from build123d import *

# Parameters (mm, degrees)
SKETCH2_R                = 3
BOSS_EXTRUDE1_DEPTH      = 20.5
BOSS_EXTRUDE1_DEPTH_BACK = 20.5
CHAMFER1_SIZE            = 0.12
CUT_EXTRUDE1_START       = -2.1
SKETCH3_R                = 3
SKETCH3_R_2              = 2.5
CUT_EXTRUDE1_DEPTH       = 0.74


with BuildPart() as part:
    # Sketch2 → Boss-Extrude1 (new body, two sides)
    with BuildSketch(Plane.XY) as boss_extrude1_sk:
        Circle(SKETCH2_R)
    extrude(amount=BOSS_EXTRUDE1_DEPTH)
    extrude(boss_extrude1_sk.sketch, amount=-BOSS_EXTRUDE1_DEPTH_BACK)

    # Chamfer1
    chamfer1_edges = [part.edges().sort_by_distance(p)[0] for p in [
        (-3, 0, -20.5),
        (-3, 0, 20.5),
    ]]
    chamfer(chamfer1_edges, length=CHAMFER1_SIZE)

    # Sketch3 → Cut-Extrude1 (cut)
    with BuildSketch(Plane.XY.offset(19.8).offset(CUT_EXTRUDE1_START)):
        Circle(SKETCH3_R)
        Circle(SKETCH3_R_2, mode=Mode.SUBTRACT)
    cut_extrude1 = extrude(amount=-CUT_EXTRUDE1_DEPTH, mode=Mode.SUBTRACT)

    # Mirror1: Cut-Extrude1 across plane
    add(cut_extrude1.mirror(Plane.XY), mode=Mode.SUBTRACT)


solid = part.part
The model under review builds one solid part; all positions refer to its coordinate system, in mm. A direction names the side the tool comes from. Round coordinates to 2 decimals unless told otherwise and drop trailing zeros. Write each loop counter-clockwise with the first axis right and the second up, starting at its lowest first coordinate (ties: lowest second). Pieces come first, ordered by that corner, then holes. Notation, with made-up numbers: M -1.5,34.5 L 11.5,34.5 A25 ccw 11.5,48.5 Z; hole C -29.5,50.5 d8. An arc over 180 degrees is marked long. Answer as CSV lines item,"result". Start each with the question number.
Q1. Wall thickness on line 1 along Z through (x, y) = (0.75, 2.45); line 2 along X through (y, z) = (-0.85, 12); line 3 along Y through (x, z) = (-0.2, -2.5): over which ranges is each line inside the solid? List them lowest first.
Q2. Clearance check with flat-ended pins moving along their axes: P1, Ø1, axis at x = 2, z = -7, coming from the +Y side; P2, Ø1.5, axis at x = -2.5, z = 15, coming from the +Y side. State where each tip first meets the part, or that it passes through.
Q3. Tool access review of faces 1 (the face through (-3, 0, -19)), 2 (the face through (-2, 2, -16.96)): name each direction out of +Z, -Z, +X, -X, +Y, -Y from which nothing blocks a thin tool from reaching the whole face with its end or side.
Q4. Consider section A-A, the plane z = 9. Give the boundary of the cut face in (x, y).
Q5. The part is to be moulded in two halves that separate along Z. For faces 3 (the face through (0, 0, -20.5)), 4 (the face through (-3, 0, 0)), 5 (the face through (0, 0, 20.5)), 6 (the face through (-2, 2, 16.96)), say which applies: +Z half, -Z half, draft (parallel to the pull), parting line (faces both ways), or undercut.
Result set:
1,line 1,"z = -20.5 to -17.7, -16.96 to 16.96, 17.7 to 20.5"
1,line 2,"x = -2.88 to 2.88"
1,line 3,"y = -2.99 to 2.99"
2,P1,"stops at y = 2.6"
2,P2,"stops at y = 2.44"
3,face 1,"+Z, -Z"
3,face 2,"none"
4,outline,"C 0,0 d6"
5,face 3,"-Z half"
5,face 4,"draft"
5,face 5,"+Z half"
5,face 6,"undercut"
